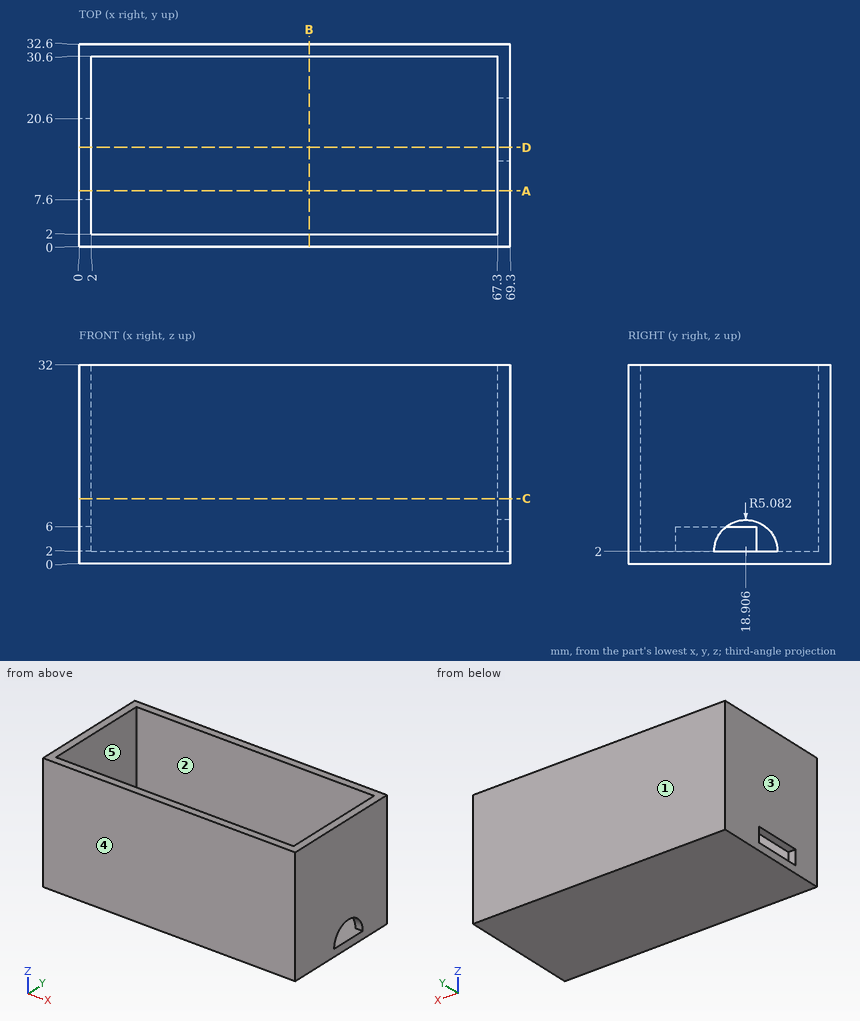
Source: three-view drawing plus pictorial views. Frame: mm from the lowest corner of the part. A direction names the side the tool comes from. Coordinates: 2 decimals unless noted, no trailing zeros. Write each loop counter-clockwise with the first axis right and the second up, starting at its lowest first coordinate (ties: lowest second). Pieces come first, ordered by that corner, then holes. Notation, with made-up numbers: (-4, 28.5) - (38, 28.5) arc R19 cw to (38, 32.5) - close; hole circle Ø7 at (-21, -15.75). An arc over 180 degrees is marked (long way). Return JSON: item names as keys, results as strings.
Item 1: Section query B-B (x = 37). Output: boundary loops of the cut face in (y, z), and give its area (3 significant figures).
Completed:
{"outline": "(0, 0) - (32.6, 0) - (32.6, 32) - (30.6, 32) - (30.6, 2) - (2, 2) - (2, 32) - (0, 32) - close", "area": "185 mm2"}
Item 2: Line query: L1, parallel to Y at x = 35.5, z = 11; L2, parallel to X at y = 26.5, z = 9.5; L3, parallel to Z at x = 25, y = 4. Output: solid intervals per line, ascending.
Completed:
{"L1": "y = 0 to 2, 30.6 to 32.6", "L2": "x = 0 to 2, 67.3 to 69.3", "L3": "z = 0 to 2"}
Item 3: Section query C-C (z = 10.5). Output: boundary loops of the cut face in (x, y).
Completed:
{"outline": "(0, 0) - (69.3, 0) - (69.3, 32.6) - (0, 32.6) - close; hole (2, 2) - (67.3, 2) - (67.3, 30.6) - (2, 30.6) - close"}
Item 4: Pin query (flat end, axial travel): pin 1 Ø8 at (x, y) = (24, 13) entering from +Z. Return the tip coordinate at first contact, or that it passes through.
Completed:
{"pin 1": "stops at z = 2"}
Item 5: Section query D-D (y = 16). Output: boundary loops of the cut face in (x, z).
Completed:
{"outline": "(0, 0) - (69.3, 0) - (69.3, 2) - (0, 2) - close; (0, 6) - (2, 6) - (2, 32) - (0, 32) - close; (67.3, 6.17) - (69.3, 6.17) - (69.3, 32) - (67.3, 32) - close"}
Item 6: Section query A-A (y = 9). Output: boundary loops of the cut face in (x, z).
Completed:
{"outline": "(0, 0) - (69.3, 0) - (69.3, 32) - (67.3, 32) - (67.3, 2) - (0, 2) - close; (0, 6) - (2, 6) - (2, 32) - (0, 32) - close"}
Item 7: Reachability of the marked faces 1 and 2 from +Z, -Z, +X, -X, +Y, -Y: full face, straight path, thin tool, end or side. Return the list, or none.
Completed:
{"face 1": "+Z, -Z, +X, -X, +Y", "face 2": "+Z"}
Item 8: Pull-direction query (Y, two-part tool) for the marked faces 3, 4 and 5; classes: +Y half, -Y half, draft (parallel to the pull), parting line (faces both ways), or undercut.
Completed:
{"face 3": "draft", "face 4": "-Y half", "face 5": "undercut"}
